```python
from build123d import *

# Parameters (mm, degrees)
ESQUISSE1_R        = 50
ESQUISSE1_R_2      = 47.5
BOSS_EXTRU_1_DEPTH = 5
BOSS_EXTRU_2_START = -2.5
BOSS_EXTRU_2_DEPTH = 2.5
CONG_2_R           = 2
BOSS_EXTRU_3_START = 2.5
BOSS_EXTRU_3_DEPTH = 2.5


with BuildPart() as part:
    # Esquisse1 → Boss.-Extru.1 (new body)
    with BuildSketch(Plane.XY):
        Circle(ESQUISSE1_R)
        Circle(ESQUISSE1_R_2, mode=Mode.SUBTRACT)
    extrude(amount=BOSS_EXTRU_1_DEPTH)

    # Esquisse2 → Boss.-Extru.2 (add)
    with BuildSketch(Plane.XY.offset(5).offset(BOSS_EXTRU_2_START)):
        with BuildLine():
            Line((-33.170016581, -34), (33.170016581, -34))
            ThreePointArc((33.170016581, -34), (0, -47.5), (-33.170016581, -34))
        make_face()
    extrude(amount=BOSS_EXTRU_2_DEPTH)

    # Congé2
    # the kernel refuses this fillet: 2 mm, written as the material it takes off along each edge
    with BuildSketch(Plane(origin=(-38.170016581, -34, 5), x_dir=(0, -1, 0), z_dir=(1, 0, 0))) as cong_2_piece_1_section:
        with BuildLine():
            CenterArc((CONG_2_R, CONG_2_R), CONG_2_R, 180, 90)
            Line((0, CONG_2_R), (0, 0))
            Line((0, 0), (CONG_2_R, 0))
        make_face()
    cong_2_piece_1 = extrude(amount=76.340033162, mode=Mode.PRIVATE)
    cong_2_piece_1 = cong_2_piece_1 & Plane(origin=(0, 0, 4.543639328), x_dir=(1, 0, 0), z_dir=(0, 0, -1)) * Cylinder(47.5, 161, mode=Mode.PRIVATE)
    add(cong_2_piece_1, mode=Mode.SUBTRACT)
    with BuildSketch(Plane(origin=(-38.170016581, -34, 2.5), x_dir=(0, 0, 1), z_dir=(1, 0, 0))) as cong_2_piece_2_section:
        with BuildLine():
            CenterArc((CONG_2_R, CONG_2_R), CONG_2_R, 180, 90)
            Line((0, CONG_2_R), (0, 0))
            Line((0, 0), (CONG_2_R, 0))
        make_face()
    cong_2_piece_2 = extrude(amount=76.340033162, mode=Mode.PRIVATE)
    cong_2_piece_2 = cong_2_piece_2 & Plane(origin=(0, 0, 2.956360666), x_dir=(1, 0, 0), z_dir=(0, 0, -1)) * Cylinder(47.5, 161, mode=Mode.PRIVATE)
    add(cong_2_piece_2, mode=Mode.SUBTRACT)

    # Esquisse3 → Boss.-Extru.3 (add)
    with BuildSketch(Plane(origin=(0, 0, 2.5), x_dir=(-1, 0, 0), z_dir=(0, 0, -1)).offset(BOSS_EXTRU_3_START)):
        with BuildLine():
            Line((-29.786742017, -37), (29.786742017, -37))
            ThreePointArc((29.786742017, -37), (0, -47.5), (-29.786742017, -37))
        make_face()
    extrude(amount=-BOSS_EXTRU_3_DEPTH)


solid = part.part
```
Can you work these out from the model? Positions are in its coordinate system, mm. Round coordinates to 2 decimals unless told otherwise and drop trailing zeros. Loops run counter-clockwise (first coordinate to the right, second up) from the corner with the lowest first, then second, coordinate; pieces in that order, holes last. Notation, with made-up numbers: (-28.75, 53) -> (-17.75, 53) arc R12 cw to (-17.75, 64) -> close; hole circle Ø9 at (-3, 62.5). An arc over 180 degrees is marked (long way). Answer in a Markdown table with one row per item.
Item 1: Suppose I cut it at A-A, the plane y = 0. List the corners of the cut face in (x, z) for me, plus the area to 3 significant figures.
Answer block:
| item | result |
|---|---|
| outline | (-50, 0) -> (-47.5, 0) -> (-47.5, 5) -> (-50, 5) -> close; (47.5, 0) -> (50, 0) -> (50, 5) -> (47.5, 5) -> close |
| area | 25.0 mm² |
Item 2: Suppose I cut it at C-C, the plane z = 0.95. List the corners of the cut face in (x, y) for me.
Answer block:
| item | result |
|---|---|
| outline | circle Ø100 at (0, 0); hole (-29.79, -37) -> (29.79, -37) arc R47.5 ccw (long way) to start |
Item 3: Suppose I cut it at D-D, the plane x = 11. List the corners of the cut face in (y, z) for me (3 decimals), plus the area to 3 significant figures.
Answer block:
| item | result |
|---|---|
| outline | (-48.775, 0) -> (-37, 0) -> (-37, 2.5) -> (-36, 2.5) arc R2 ccw to (-34.146, 3.75) arc R2 ccw to (-36, 5) -> (-48.775, 5) -> close; (46.209, 0) -> (48.775, 0) -> (48.775, 5) -> (46.209, 5) -> close |
| area | 77.6 mm² |
Item 4: We'd pull the mould along Y, two halves only. Please class faces 1 (the flat face through (0, -41, 0)), 2 (the cylindrical face through (47.69, 15.02, 2.46)), 3 (the flat face through (0, -37, 1)): released by +Y, released by -Y, zero draft, split by the parting line, or undercut.
Answer block:
| item | result |
|---|---|
| face 1 | zero draft |
| face 2 | split by the parting line |
| face 3 | undercut |
Item 5: If I drill on probe 1 along Y at (x, z) = (0, 1.95); probe 2 along Y at (x, z) = (-25.5, 4.8); probe 3 along X at (y, z) = (-4.5, 3.95), over which ranges is the centre line in solid material (lowest first)?
Answer block:
| item | result |
|---|---|
| probe 1 | -50 to -37, 47.5 to 50 |
| probe 2 | -43.01 to -35.13, 40.07 to 43.01 |
| probe 3 | -49.8 to -47.29, 47.29 to 49.8 |
Item 6: Will these pins go through, and if not, where does the flat tip stop? P1, Ø1, axis at x = 2.5, y = -34, coming from the +Z side; P2, Ø1, axis at y = -19.5, z = 2, coming from the -X side; P3, Ø2, axis at x = -6, z = 1.5, coming from the +Y side.
Answer block:
| item | result |
|---|---|
| P1 | z = 4.32 |
| P2 | x = -46.25 |
| P3 | y = 49.75 |
Item 7: Suppose I cut it at B-B, the plane x = 0. List the corners of the cut face in (y, z) for me, plus the area to 3 significant figures.
Answer block:
| item | result |
|---|---|
| outline | (-50, 0) -> (-37, 0) -> (-37, 2.5) -> (-36, 2.5) arc R2 ccw to (-34.15, 3.75) arc R2 ccw to (-36, 5) -> (-50, 5) -> close; (47.5, 0) -> (50, 0) -> (50, 5) -> (47.5, 5) -> close |
| area | 83.4 mm² |
